from build123d import *

# Parameters (mm, degrees)
SKETCH_13_W         = 7
SKETCH_13_H         = 1
CUT_EXTRUDE_9_DEPTH = 1.8
FILLET_1_R          = 0.1
CHAMFER_1_SIZE      = 0.75


with BuildPart() as part:
    # Sketch 1 → Revolve 1 (revolve)
    with BuildSketch(Plane.XY, mode=Mode.PRIVATE) as revolve_1_sk:
        with BuildLine():
            Line((2, 91.44931314), (3.5, 91.44931314))
            ThreePointArc((3.5, 91.44931314), (2.438021098, 93.318621459), (0.5, 94.24931314))
            Line((0.5, 94.24931314), (0, 94.24931314))
            Line((0, 94.24931314), (0, 84.24931314))
            Line((0, 84.24931314), (2, 84.24931314))
            Line((2, 84.24931314), (2, 91.44931314))
        make_face()
    revolve(revolve_1_sk.sketch.rotate(Axis((0, 125.763182898, 0), (0, -1, 0)), 180), axis=Axis((0, 125.763182898, 0), (0, -1, 0)))

    # Sketch 13 → Cut-Extrude 9 (cut)
    with BuildSketch(Plane(origin=(0, 94.24931314, 0), x_dir=(-1, 0, 0), z_dir=(0, 1, 0))):
        Rectangle(SKETCH_13_W, SKETCH_13_H)
    extrude(amount=-CUT_EXTRUDE_9_DEPTH, mode=Mode.SUBTRACT)

    # Fillet 1
    fillet_1_edges = [part.edges().sort_by_distance(p)[0] for p in [
        (3.5, 91.44931314, 0),
    ]]
    fillet(fillet_1_edges, radius=FILLET_1_R)

    # Chamfer 1
    chamfer_1_edges = [part.edges().sort_by_distance(p)[0] for p in [
        (2, 84.24931314, 0),
    ]]
    chamfer(chamfer_1_edges, length=CHAMFER_1_SIZE)


solid = part.part
The model under review builds one solid part; all positions refer to its coordinate system, in mm. A direction names the side the tool comes from. Give positions to 0.01 mm unless a question says otherwise; leave off trailing zeros. Write each loop counter-clockwise with the first axis right and the second up, starting at its lowest first coordinate (ties: lowest second). Pieces come first, ordered by that corner, then holes. Notation, with made-up numbers: M 42,23.25 L 51,23.25 A8 cw 51,28.25 Z; hole C 0.5,7.5 d1. An arc over 180 degrees is marked long. One line per question, with ' | ' between items. Start each with the question number.
Item 1: For faces 1 (the flat face through (0, 93, 0.5)), 2 (the flat face through (0, 84.249, 0)), list the 3-axis set-ups (+Z, -Z, +X, -X, +Y, -Y) from which the entire face can be reached by the end or side of a thin tool; tool diameter is ignored.
Item 2: For pin 1 (2 mm diameter, centred on y = 90, z = -2, fed in from -X); pin 2 (0.5 mm diameter, centred on x = -1, y = 93.5, fed in from -Z); pin 3 (0.5 mm diameter, centred on x = -1.5, y = 93.5, fed in from +Z), all flat-tipped, find the tip position at first contact; note any pin that passes through.
Item 3: Wall thickness on line 1 (Z direction, x = 2.25, y = 93.25); line 2 (Z direction, x = 0, y = 93.75); line 3 (Z direction, x = 1.5, y = 87.25): over which ranges is each line inside the solid? List them lowest first. Write a range as from..to.
Item 4: Draft analysis for pull direction Z (two halves, no side actions). For faces 3 (the cylindrical face through (0, 88, 2)), 4 (the flat face through (0, 93, -0.5)), 5 (the flat face through (0, 92.449, 0)), 6 (the flat face through (1, 91.449, 2)), state which applies: released by +Z, released by -Z, zero draft, split by the parting line, or undercut.
Item 5: We need section A-A on y = 85.25. Write out the cut boundary in (x, z).
Results found:
1) face 1: +X, -X, +Y | face 2: +Z, -Z, +X, -X, -Y
2) pin 1: stops at x = -1.73 | pin 2: stops at z = -2.32 | pin 3: stops at z = 2.06
3) line 1: z = -1.11..-0.5, 0.5..1.11 | line 2: z = -1.87..-0.5, 0.5..1.87 | line 3: z = -1.32..1.32
4) face 3: split by the parting line | face 4: undercut | face 5: undercut | face 6: zero draft
5) outline: C 0,0 d4
